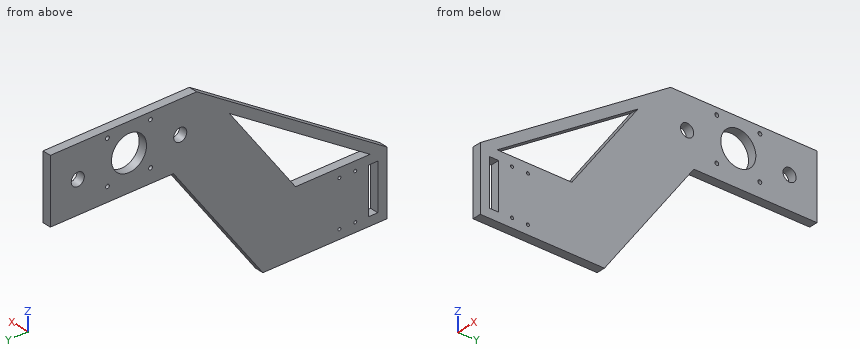
```python
from build123d import *

# Parameters (mm, degrees)
SKETCH1_R           = 7.15
SKETCH1_R_2         = 19.15
SKETCH1_W           = 50.4
SKETCH1_H           = 9.9
BOSS_EXTRUDE1_DEPTH = 9.5
M4_TAPPED_HOLE1_D   = 3.3
M5_TAPPED_HOLE2_D   = 4.2


with BuildPart() as part:
    # Sketch1 → Boss-Extrude1 (new body)
    with BuildSketch(Plane(origin=(0, 0, 0), x_dir=(0, 0, -1), z_dir=(1, 0, 0))):
        Polygon((0, 0), (70, 0), (70, 135.667122158), (-64.5, 233.385504136), (-64.5, 368), (-134.5, 368), (-134.5, 208), align=None)
        with Locations((-99.5, 338)):
            Circle(SKETCH1_R, mode=Mode.SUBTRACT)
        with Locations((-99.5, 226)):
            Circle(SKETCH1_R, mode=Mode.SUBTRACT)
        with Locations((-103.5, 282)):
            Circle(SKETCH1_R_2, mode=Mode.SUBTRACT)
        Polygon((-99.5, 172.289806742), (0, 100), (0, 18.416200794), align=None, mode=Mode.SUBTRACT)
        with Locations((35, 15.05)):
            Rectangle(SKETCH1_W, SKETCH1_H, mode=Mode.SUBTRACT)
    extrude(amount=BOSS_EXTRUDE1_DEPTH)

    # M4 Tapped Hole1 (through all)
    with Locations(Plane(origin=(9.5, 0, 0), x_dir=(0, 0, -1), z_dir=(1, 0, 0))):
        with Locations((10, 34.7), (10, 52), (60, 52), (60, 34.7)):
            Hole(M4_TAPPED_HOLE1_D / 2)

    # M5 Tapped Hole2 (through all)
    with Locations(Plane(origin=(9.5, 0, 0), x_dir=(0, 0, -1), z_dir=(1, 0, 0))):
        with Locations((-127.05, 305.55), (-79.95, 305.55), (-79.95, 258.45), (-127.05, 258.45)):
            Hole(M5_TAPPED_HOLE2_D / 2)


solid = part.part
```
Design review of the part built by this model. Coordinates are the model's own, in mm. Coordinates: 2 decimals unless noted, no trailing zeros. Write each loop counter-clockwise with the first axis right and the second up, starting at its lowest first coordinate (ties: lowest second). Pieces come first, ordered by that corner, then holes.
1) Add section B-B (y = 338). Write out the cut boundary in (x, z), plus the area to 3 significant figures.
2) To check wall thickness, follow L1, parallel to Z at x = 3, y = 338; L2, parallel to Z at x = 7.5, y = 258.45; L3, parallel to Y at x = 6, z = -10. State the ranges of each line that lie inside material, in increasing order.
3) Add section C-C (z = 70.5). Write out the cut boundary in (x, y).
4) Add section A-A (x = 3.5). State how many separate pieces and enclosed holes the cut face has, plus the area to 3 significant figures.
5) Insertion check: pin 1 (3 mm diameter, centred on x = 1, y = 331, fed in from -Z); pin 2 (5 mm diameter, centred on x = 6.5, y = 166, fed in from +Z); pin 3 (3 mm diameter, centred on x = 6.5, z = 95.5, fed in from -Y). Each pin has a flat end and moves straight along its axis. Give the tip position at first contact, or say it passes through.
Check result:
1. outline: (0, 64.5) - (9.5, 64.5) - (9.5, 92.35) - (0, 92.35) - close; (0, 106.65) - (9.5, 106.65) - (9.5, 134.5) - (0, 134.5) - close
1. area: 529 mm2
2. L1: z = 64.5 to 92.35, 106.65 to 134.5
2. L2: z = 64.5 to 77.85, 82.05 to 124.95, 129.15 to 134.5
2. L3: y = 0 to 10.1, 20 to 33.05, 36.35 to 50.35, 53.65 to 179.26
3. outline: (0, 109.03) - (9.5, 109.03) - (9.5, 127.44) - (0, 127.44) - close; (0, 151.22) - (9.5, 151.22) - (9.5, 368) - (0, 368) - close
4. separate pieces: 1
4. enclosed holes: 13
4. area: 30,500 mm2
5. pin 1: stops at z = 64.5
5. pin 2: stops at z = 108.96
5. pin 3: stops at y = 145.37
